Part model, mm, in its own coordinate system. Give positions to 0.01 mm unless a question says otherwise; leave off trailing zeros. Write each loop counter-clockwise with the first axis right and the second up, starting at its lowest first coordinate (ties: lowest second). Pieces come first, ordered by that corner, then holes.
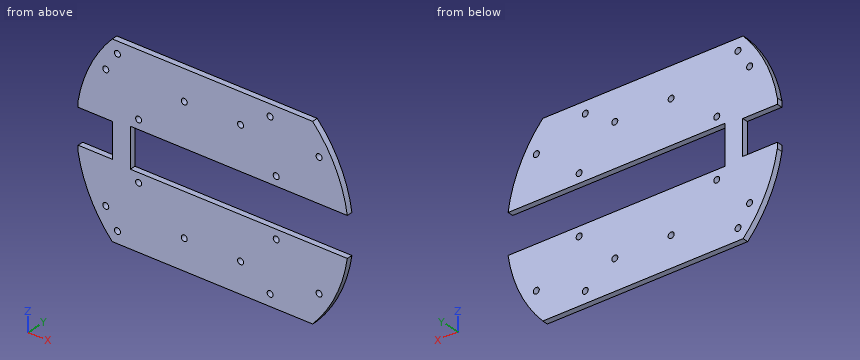
```python
from build123d import *

# Parameters (mm, degrees)
SKETCH1_R           = 1.651
BOSS_EXTRUDE1_DEPTH = 3.175
SKETCH2_W           = 19.05
SKETCH2_H           = 19.05
CUT_EXTRUDE1_DEPTH  = 3.175


with BuildPart() as part:
    # Sketch1 → Boss-Extrude1 (new body)
    with BuildSketch(Plane(origin=(0, 0, 0), x_dir=(1, 0, 0), z_dir=(0, 1, 0))):
        with BuildLine():
            Line((-73.916912814, 12.7), (-73.916912814, -12.7))
            ThreePointArc((-73.916912814, -12.7), (-67.281551776, -33.138991997), (-55.122759171, -50.857461806))
            Line((-55.122759171, -50.857461806), (55.122759171, -50.857461806))
            ThreePointArc((55.122759171, -50.857461806), (67.702114955, -32.271095901), (74.219053989, -10.795))
            Line((74.219053989, -10.795), (-45.158734092, -10.795))
            Line((-45.158734092, -10.795), (-45.158734092, 10.795))
            Line((-45.158734092, 10.795), (74.219053989, 10.795))
            ThreePointArc((74.219053989, 10.795), (67.702114955, 32.271095901), (55.122759171, 50.857461806))
            Line((55.122759171, 50.857461806), (-55.122759171, 50.857461806))
            ThreePointArc((-55.122759171, 50.857461806), (-67.281551776, 33.138991997), (-73.916912814, 12.7))
        make_face()
        with Locations(Location((31.75, 44.507461806, 0), (0, 0, 270))):
            Circle(SKETCH1_R, mode=Mode.SUBTRACT)
        with Locations(Location((35.105265908, 15.875, 0), (0, 0, 270))):
            Circle(SKETCH1_R, mode=Mode.SUBTRACT)
        with Locations(Location((35.105265908, -15.875, 0), (0, 0, 270))):
            Circle(SKETCH1_R, mode=Mode.SUBTRACT)
        with Locations(Location((-40.594426833, -15.875, 0), (0, 0, 270))):
            Circle(SKETCH1_R, mode=Mode.SUBTRACT)
        with Locations(Location((-40.594426833, 15.875, 0), (0, 0, 270))):
            Circle(SKETCH1_R, mode=Mode.SUBTRACT)
        with Locations(Location((31.75, -44.507461806, 0), (0, 0, 270))):
            Circle(SKETCH1_R, mode=Mode.SUBTRACT)
        with Locations(Location((-52.26766059, -44.507461806, 0), (0, 0, 270))):
            Circle(SKETCH1_R, mode=Mode.SUBTRACT)
        with Locations(Location((-52.26766059, 44.507461806, 0), (0, 0, 270))):
            Circle(SKETCH1_R, mode=Mode.SUBTRACT)
        with Locations(Location((-58.676912814, 34.29, 0), (0, 0, 270))):
            Circle(SKETCH1_R, mode=Mode.SUBTRACT)
        with Locations(Location((-15.496912814, 34.29, 0), (0, 0, 270))):
            Circle(SKETCH1_R, mode=Mode.SUBTRACT)
        with Locations(Location((-15.496912814, -34.29, 0), (0, 0, 270))):
            Circle(SKETCH1_R, mode=Mode.SUBTRACT)
        with Locations(Location((-58.676912814, -34.29, 0), (0, 0, 270))):
            Circle(SKETCH1_R, mode=Mode.SUBTRACT)
        with Locations(Location((15.496912814, -34.29, 0), (0, 0, 90))):
            Circle(SKETCH1_R, mode=Mode.SUBTRACT)
        with Locations(Location((58.676912814, -34.29, 0), (0, 0, 90))):
            Circle(SKETCH1_R, mode=Mode.SUBTRACT)
        with Locations(Location((58.676912814, 34.29, 0), (0, 0, 90))):
            Circle(SKETCH1_R, mode=Mode.SUBTRACT)
        with Locations(Location((15.496912814, 34.29, 0), (0, 0, 90))):
            Circle(SKETCH1_R, mode=Mode.SUBTRACT)
    extrude(amount=BOSS_EXTRUDE1_DEPTH)

    # Sketch2 → Cut-Extrude1 (cut)
    with BuildSketch(Plane(origin=(0, 3.175, 0), x_dir=(1, 0, 0), z_dir=(0, 1, 0))):
        with Locations((-64.391912814, 0)):
            Rectangle(SKETCH2_W, SKETCH2_H)
    extrude(amount=-CUT_EXTRUDE1_DEPTH, mode=Mode.SUBTRACT)


solid = part.part
```
1) Saw through at B-B, the plane x = -26. Write the cut outline in (y, z) (3 decimals), then the cut area to 3 significant figures.
Answers follow:
outline: (0, -50.857) - (3.175, -50.857) - (3.175, -10.795) - (0, -10.795) - close; (0, 10.795) - (3.175, 10.795) - (3.175, 50.857) - (0, 50.857) - close
area: 254 mm2
2) Saw through at C-C, the plane z = -34.29. Write the cut outline in (x, y) (3 decimals), then the cut area to 3 significant figures.
Answers follow:
outline: (-66.702, 0) - (-60.328, 0) - (-60.328, 3.175) - (-66.702, 3.175) - close; (-57.026, 0) - (-17.148, 0) - (-17.148, 3.175) - (-57.026, 3.175) - close; (-13.846, 0) - (13.846, 0) - (13.846, 3.175) - (-13.846, 3.175) - close; (17.148, 0) - (57.026, 0) - (57.026, 3.175) - (17.148, 3.175) - close; (60.328, 0) - (66.702, 0) - (66.702, 3.175) - (60.328, 3.175) - close
area: 382 mm2
3) Wall check: L1, parallel to Z at x = 51, y = 0.7 (3 decimals); L2, parallel to Z at x = 36.5, y = 0.75 (3 decimals); L3, parallel to X at y = 0.7, z = -34. Give the ranges that are in metal, low to high.
Answers follow:
L1: z = -50.857 to -10.795, 10.795 to 50.857
L2: z = -50.857 to -16.758, -14.992 to -10.795, 10.795 to 14.992, 16.758 to 50.857
L3: x = -66.85 to -60.3, -57.05 to -17.12, -13.87 to 13.87, 17.12 to 57.05, 60.3 to 66.85
4) Saw through at A-A, the plane x = 31.75. Write the cut outline in (y, z) (3 decimals), then the cut area to 3 significant figures.
Answers follow:
outline: (0, -50.857) - (3.175, -50.857) - (3.175, -46.158) - (0, -46.158) - close; (0, -42.856) - (3.175, -42.856) - (3.175, -10.795) - (0, -10.795) - close; (0, 10.795) - (3.175, 10.795) - (3.175, 42.856) - (0, 42.856) - close; (0, 46.158) - (3.175, 46.158) - (3.175, 50.857) - (0, 50.857) - close
area: 233 mm2
5) Pin check, flat tips, straight feed: pin 1 Ø1.5 at (y, z) = (2, 38) entering from +X; pin 2 Ø1 at (y, z) = (1.5, 0.5) entering from -X; pin 3 Ø2 at (x, z) = (15.5, -34.29) entering from -Y; pin 4 Ø1 at (y, z) = (2, 3) entering from +X. Stop position of each tip, or through.
Answers follow:
pin 1: stops at x = 65.1
pin 2: stops at x = -54.87
pin 3: passes through
pin 4: stops at x = -45.16
6) Saw through at D-D, the plane y = 0.8. Count the separate pieces of the cut face and the enclosed holes in it, then the cut area to 3 significant figures.
Answers follow:
separate pieces: 1
enclosed holes: 16
area: 10,900 mm2
